from build123d import *

# Parameters (mm, degrees)
F0_W     = 210
F0_H     = 147
F1_DEPTH = 3
F2_R     = 4
F3_DEPTH = 15
F4_R     = 1.75
F5_DEPTH = 25


with BuildPart() as f1:
    # F0 (on Top) → F1 (new body)
    with BuildSketch(Plane.XY):
        with Locations((105, -73.5)):
            Rectangle(F0_W, F0_H)
    extrude(amount=F1_DEPTH)

    # F2 (on face) → F3 (join)
    with BuildSketch(Plane.XY.offset(3)):
        with Locations((10, -35)):
            Circle(F2_R)
        with Locations((184, -35)):
            Circle(F2_R)
        with Locations((184, -137)):
            Circle(F2_R)
        with Locations((10, -137)):
            Circle(F2_R)
    extrude(amount=F3_DEPTH)

    # F4 (on face) → F5 (cut)
    with BuildSketch(Plane.XY.offset(3)):
        with Locations((5, -5)):
            Circle(F4_R)
        with Locations((145, -5)):
            Circle(F4_R)
    extrude(amount=-F5_DEPTH, mode=Mode.SUBTRACT)


solid = f1.part
Design review of the part built by this model. Coordinates are the model's own, in mm. A direction names the side the tool comes from. Coordinates: 2 decimals unless noted, no trailing zeros. Loops run counter-clockwise (first coordinate to the right, second up) from the corner with the lowest first, then second, coordinate; pieces in that order, holes last. Notation, with made-up numbers: (37.25, 65.25) -> (56.25, 65.25) arc R13 ccw to (56.25, 81.25) -> close; hole circle Ø5 at (5, -6.75). An arc over 180 degrees is marked (long way). Use a Markdown table: item, result. Add a question column.
Item 1: Clearance check with flat-ended pins moving along their axes: P1, Ø1, axis at y = -31, z = 7.5, coming from the -X side; P2, Ø3, axis at x = 53.5, y = -24, coming from the +Z side; P3, Ø3, axis at x = 5, y = -5, coming from the +Z side; P4, Ø3, axis at x = 67.5, z = 2, coming from the +Y side. State where each tip first meets the part, or that it passes through.
Item 2: We need section B-B, the plane x = 184. Write out the cut boundary in (y, z).
Item 3: We need section A-A, the plane z = 10. Write out the cut boundary in (x, y), and give its area (3 significant figures).
Item 4: The part is to be moulded in two halves that separate along X. For faces 3 (the flat face through (104, -72, 0)), 4 (the cylindrical face through (9.479, -133.034, 10.395)), say which applies: +X half, -X half, draft (parallel to the pull), parting line (faces both ways), or undercut.
Item 5: Machinability: for faces 1 (the cylindrical face through (187.815, -33.799, 10.395)), 2 (the flat face through (184, -35, 18)), which of the approach directions +Z, -Z, +X, -X, +Y, -Y give a long, thin tool a straight path to every point of the face, cutting with its end or side? Answer none if there is none.
Item 6: We need section D-D, the plane y = -97.5. Write out the cut boundary in (x, z).
Item 7: We need section C-C, the plane y = -35. Write out the cut boundary in (x, z), and give its area (3 significant figures).
Item 8: Wall thickness on L1, parallel to Y at x = 5, z = 2; L2, parallel to Z at x = 36.5, y = -90: over which ranges is each line inside the solid? List them lowest first. Write a range as from..to.
Numbers:
| question | item | result |
|---|---|---|
| 1 | P1 | stops at x = 8.06 |
| 1 | P2 | stops at z = 3 |
| 1 | P3 | passes through |
| 1 | P4 | stops at y = 0 |
| 2 | outline | (-147, 0) -> (0, 0) -> (0, 3) -> (-31, 3) -> (-31, 18) -> (-39, 18) -> (-39, 3) -> (-133, 3) -> (-133, 18) -> (-141, 18) -> (-141, 3) -> (-147, 3) -> close |
| 3 | outline | circle Ø8 at (10, -137); circle Ø8 at (10, -35); circle Ø8 at (184, -137); circle Ø8 at (184, -35) |
| 3 | area | 201 mm^2 |
| 4 | face 3 | draft |
| 4 | face 4 | undercut |
| 5 | face 1 | +Z |
| 5 | face 2 | +Z, +X, -X, +Y, -Y |
| 6 | outline | (0, 0) -> (210, 0) -> (210, 3) -> (0, 3) -> close |
| 7 | outline | (0, 0) -> (210, 0) -> (210, 3) -> (188, 3) -> (188, 18) -> (180, 18) -> (180, 3) -> (14, 3) -> (14, 18) -> (6, 18) -> (6, 3) -> (0, 3) -> close |
| 7 | area | 870 mm^2 |
| 8 | L1 | y = -147..-6.75, -3.25..0 |
| 8 | L2 | z = 0..3 |
